Could you check a few things on this model? Use its own coordinates, in mm. A direction names the side the tool comes from. Round coordinates to 2 decimals unless told otherwise and drop trailing zeros. Write each loop counter-clockwise with the first axis right and the second up, starting at its lowest first coordinate (ties: lowest second). Pieces come first, ordered by that corner, then holes. Notation, with made-up numbers: (17.25, 24.5) - (30.25, 24.5) arc R32 ccw to (30.25, 62.5) - close; hole circle Ø8 at (56, -3.5). An arc over 180 degrees is marked (long way). Put each result on its own line as item: value.
from build123d import *

# Parameters (mm, degrees)
F0_W     = 27
F0_H     = 15.9
F0_W_2   = 15.9
F0_H_2   = 27
F0_W_3   = 3
F0_H_3   = 3
F1_DEPTH = 21.9
F2_DEPTH = 51.8
F3_R     = 7.95
F6_DEPTH = 30
F7_DEPTH = 30
F4_R     = 7.9
F8_DEPTH = 30


with BuildPart() as f1:
    # F0 (on Front) → F1 (new body)
    with BuildSketch(Plane.XZ):
        with BuildLine():
            Line((-34.3576915575, 15.9), (-42.3076915575, 15.9))
            Line((-42.3076915575, 15.9), (-42.3076915575, 7.9499999931))
            ThreePointArc((-42.3076915575, 7.9499999931), (-39.9791904704, 13.571498908), (-34.3576915575, 15.9))
        make_face()
        with BuildLine():
            ThreePointArc((-34.3576915575, 15.9), (-39.9791904704, 13.571498908), (-42.3076915575, 7.9499999931))
            ThreePointArc((-42.3076915575, 7.9499999931), (-39.9791904655, 2.3285010871), (-34.3576915575, 0))
            ThreePointArc((-34.3576915575, 0), (-28.7361926471, 2.3285010896), (-26.4076915575, 7.95))
            ThreePointArc((-26.4076915575, 7.95), (-28.7361926471, 13.5714989104), (-34.3576915575, 15.9))
        make_face()
        Polygon((-42.3076915575, 18.9), (-42.3076915575, 45.9), (-26.4076915575, 45.9), (-26.4076915575, 18.9), (-23.4076915575, 18.9), (-23.4076915575, 48.9), (-45.3076915575, 48.9), (-45.3076915575, 18.9), align=None)
        with Locations((-9.9076915575, 7.95)):
            Rectangle(F0_W, F0_H)
        with Locations((-34.3576915575, 32.4)):
            Rectangle(F0_W_2, F0_H_2)
        with BuildLine():
            ThreePointArc((-34.3576915575, 0), (-39.9791904655, 2.3285010871), (-42.3076915575, 7.9499999931))
            Line((-42.3076915575, 7.9499999931), (-42.3076915575, 0))
            Line((-42.3076915575, 0), (-34.3576915575, 0))
        make_face()
        with BuildLine():
            Line((-26.4076915575, 0), (-26.4076915575, 7.95))
            ThreePointArc((-26.4076915575, 7.95), (-28.7361926471, 2.3285010896), (-34.3576915575, 0))
            Line((-34.3576915575, 0), (-26.4076915575, 0))
        make_face()
        with BuildLine():
            Line((-26.4076915575, 7.95), (-26.4076915575, 15.9))
            Line((-26.4076915575, 15.9), (-34.3576915575, 15.9))
            ThreePointArc((-34.3576915575, 15.9), (-28.7361926471, 13.5714989104), (-26.4076915575, 7.95))
        make_face()
        Polygon((6.5923084425, 18.9), (-23.4076915575, 18.9), (-23.4076915575, 15.9), (3.5923084425, 15.9), (3.5923084425, 0), (-23.4076915575, 0), (-23.4076915575, -3), (6.5923084425, -3), align=None)
        Polygon((-26.4076915575, 18.9), (-42.3076915575, 18.9), (-42.3076915575, 15.9), (-34.3576915575, 15.9), (-26.4076915575, 15.9), align=None)
        Polygon((-23.4076915575, 15.9), (-26.4076915575, 15.9), (-26.4076915575, 7.95), (-26.4076915575, 0), (-23.4076915575, 0), align=None)
        Polygon((-42.3076915575, 15.9), (-42.3076915575, 18.9), (-45.3076915575, 18.9), (-45.3076915575, -3), (-23.4076915575, -3), (-23.4076915575, 0), (-26.4076915575, 0), (-34.3576915575, 0), (-42.3076915575, 0), (-42.3076915575, 7.9499999931), align=None)
        with Locations((-24.9076915575, 17.4)):
            Rectangle(F0_W_3, F0_H_3)
    extrude(amount=F1_DEPTH)

    # F0 (on Front) → F2 (join)
    with BuildSketch(Plane.XZ):
        Polygon((-42.3076915575, 15.9), (-42.3076915575, 18.9), (-45.3076915575, 18.9), (-45.3076915575, -3), (-23.4076915575, -3), (-23.4076915575, 0), (-26.4076915575, 0), (-34.3576915575, 0), (-42.3076915575, 0), (-42.3076915575, 7.9499999931), align=None)
        with BuildLine():
            ThreePointArc((-34.3576915575, 15.9), (-39.9791904704, 13.571498908), (-42.3076915575, 7.9499999931))
            ThreePointArc((-42.3076915575, 7.9499999931), (-39.9791904655, 2.3285010871), (-34.3576915575, 0))
            ThreePointArc((-34.3576915575, 0), (-28.7361926471, 2.3285010896), (-26.4076915575, 7.95))
            ThreePointArc((-26.4076915575, 7.95), (-28.7361926471, 13.5714989104), (-34.3576915575, 15.9))
        make_face()
        Polygon((-26.4076915575, 18.9), (-42.3076915575, 18.9), (-42.3076915575, 15.9), (-34.3576915575, 15.9), (-26.4076915575, 15.9), align=None)
        Polygon((-23.4076915575, 15.9), (-26.4076915575, 15.9), (-26.4076915575, 7.95), (-26.4076915575, 0), (-23.4076915575, 0), align=None)
        with Locations((-24.9076915575, 17.4)):
            Rectangle(F0_W_3, F0_H_3)
        with BuildLine():
            Line((-26.4076915575, 7.95), (-26.4076915575, 15.9))
            Line((-26.4076915575, 15.9), (-34.3576915575, 15.9))
            ThreePointArc((-34.3576915575, 15.9), (-28.7361926471, 13.5714989104), (-26.4076915575, 7.95))
        make_face()
        with BuildLine():
            Line((-34.3576915575, 15.9), (-42.3076915575, 15.9))
            Line((-42.3076915575, 15.9), (-42.3076915575, 7.9499999931))
            ThreePointArc((-42.3076915575, 7.9499999931), (-39.9791904704, 13.571498908), (-34.3576915575, 15.9))
        make_face()
        with BuildLine():
            ThreePointArc((-34.3576915575, 0), (-39.9791904655, 2.3285010871), (-42.3076915575, 7.9499999931))
            Line((-42.3076915575, 7.9499999931), (-42.3076915575, 0))
            Line((-42.3076915575, 0), (-34.3576915575, 0))
        make_face()
        with BuildLine():
            Line((-26.4076915575, 0), (-26.4076915575, 7.95))
            ThreePointArc((-26.4076915575, 7.95), (-28.7361926471, 2.3285010896), (-34.3576915575, 0))
            Line((-34.3576915575, 0), (-26.4076915575, 0))
        make_face()
    extrude(amount=F2_DEPTH)

    # F3 (on face) → F6 (cut)
    with BuildSketch(Plane.XZ.offset(51.8)):
        with Locations((-34.3576915575, 7.95)):
            Circle(F3_R)
    extrude(amount=-F6_DEPTH, mode=Mode.SUBTRACT)

    # F5 (on face) → F7 (cut)
    with BuildSketch(Plane.YZ.offset(6.5923084425)):
        with BuildLine():
            ThreePointArc((-3, 7.95), (-5.3285010896, 13.5714989104), (-10.95, 15.9))
            ThreePointArc((-10.95, 15.9), (-16.5714989104, 13.5714989104), (-18.9, 7.95))
            ThreePointArc((-18.9, 7.95), (-16.5714989104, 2.3285010896), (-10.95, 0))
            ThreePointArc((-10.95, 0), (-5.3285010896, 2.3285010896), (-3, 7.95))
        make_face()
    extrude(amount=-F7_DEPTH, mode=Mode.SUBTRACT)

    # F4 (on face) → F8 (cut)
    with BuildSketch(Plane.XY.offset(48.9)):
        with Locations((-34.3576915575, -10.9)):
            Circle(F4_R)
    extrude(amount=-F8_DEPTH, mode=Mode.SUBTRACT)


solid = f1.part
(1) Imagine slicing it at A-A, the plane x = -15.5. List the corners of the cut face in (y, z) for me.
Values found:
outline: (-21.9, -3) - (0, -3) - (0, 18.9) - (-21.9, 18.9) - close; hole circle Ø15.9 at (-10.95, 7.95)
(2) Please list where these lines run through material, in increasing order: probe 1 along Z at (x, y) = (-34.5, -30.5); probe 2 along X at (y, z) = (-31, 7); probe 3 along Y at (x, z) = (-34, 22). Write a range as from..to.
Values found:
probe 1: z = -3..0, 15.9..18.9
probe 2: x = -45.31..-42.25, -26.46..-23.41
probe 3: y = -21.9..-18.79, -3.01..0
(3) Imagine slicing it at B-B, the plane y = -41. List the corners of the cut face in (x, z) for me, then the cut area to 3 significant figures.
Values found:
outline: (-45.31, -3) - (-23.41, -3) - (-23.41, 18.9) - (-45.31, 18.9) - close; hole circle Ø15.9 at (-34.36, 7.95)
area: 281 mm^2
(4) Imagine slicing it at D-D, the plane y = -4. List the corners of the cut face in (x, z) for me, then the cut area to 3 significant figures.
Values found:
outline: (-45.31, -3) - (6.59, -3) - (6.59, 4.09) - (-23.41, 4.09) - (-23.41, 11.81) - (6.59, 11.81) - (6.59, 18.9) - (-23.41, 18.9) - (-23.41, 48.9) - (-30.51, 48.9) - (-30.51, 18.9) - (-38.2, 18.9) - (-38.2, 48.9) - (-45.31, 48.9) - close
area: 1,330 mm^2
(5) If we mould it in two halves opening along Y, with no side actions, what happens to faces 6 (the face through (-23.408, -11, 8)), 7 (the face through (-45.308, -20, 18)), 8 (the face through (-25, 0, 18)), 9 (the face through (-42, -51.8, 13))? For each: pulls with the +Y half, pulls with the -Y half, needs draft (parallel to the pull), parting line crosses it, or undercut.
Values found:
face 6: undercut
face 7: needs draft
face 8: pulls with the +Y half
face 9: pulls with the -Y half
(6) For faces 1 (the face through (-23.408, -37, 8)), 2 (the face through (-23.408, -11, 34)), 3 (the face through (-34, -21.8, 8)), 4 (the face through (-42.25, -10.55, 34.11)), 5 (the face through (-34, -37, 18.9)), which set-ups out of +Z, -Z, +X, -X, +Y, -Y let a thin tool reach every point of the face, with its end or its side?
Values found:
face 1: +Z, -Z, +X, -Y
face 2: +Z, +X, +Y, -Y
face 3: -Y
face 4: +Z
face 5: +Z, +X, -X, -Y
(7) Imagine slicing it at C-C, the plane z = 20. List the corners of the cut face in (x, y) for me, then the cut area to 3 significant figures.
Values found:
outline: (-45.31, -21.9) - (-23.41, -21.9) - (-23.41, 0) - (-45.31, 0) - close; hole circle Ø15.8 at (-34.36, -10.9)
area: 284 mm^2
(8) I'm going to push flat-ended pins straight in: pin 1 (8 mm diameter, centred on x = -33.5, y = -10.5, fed in from +Z); pin 2 (10 mm diameter, centred on x = -22.5, y = -23, fed in from -Z); pin 3 (17.5 mm diameter, centred on y = -43.5, z = 12, fed in from +X); pin 4 (11 mm diameter, centred on x = -16, z = 8, fed in from -Y). Where does each tip first touch, or does it pass through?
Values found:
pin 1: stops at z = 18.9
pin 2: stops at z = -3
pin 3: stops at x = -23.41
pin 4: stops at y = -21.9
